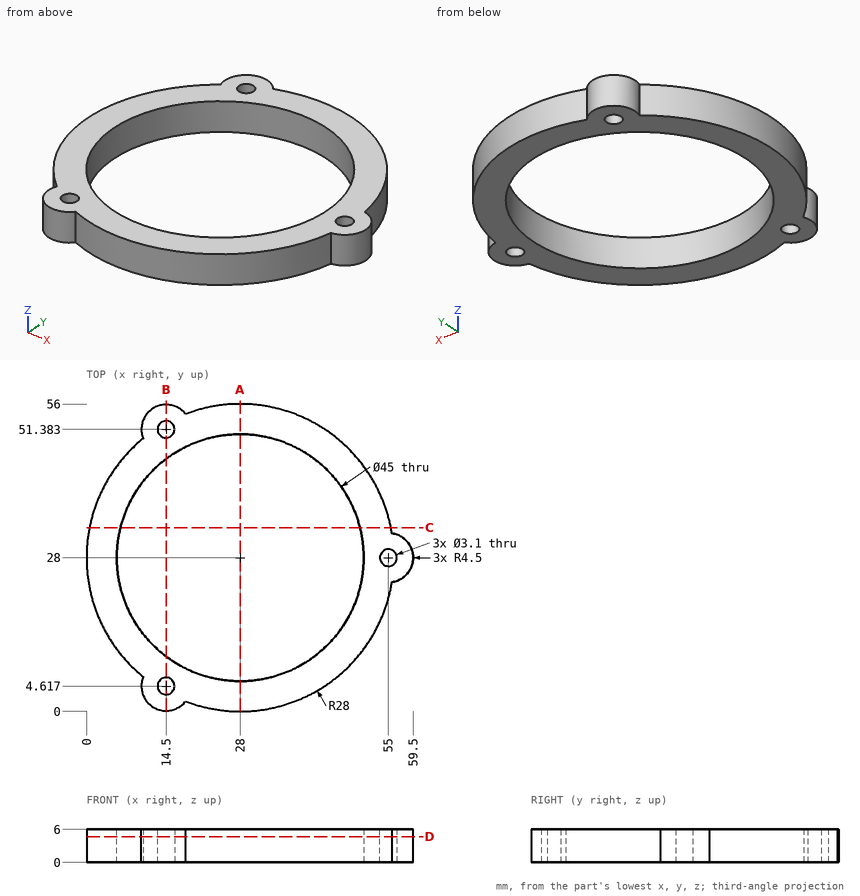
The figure shows three views and two pictorial views of one solid part (mm, origin at its lowest corner). Answer the questions. Give positions to 0.01 mm unless a question says otherwise; leave off trailing zeros. Write each loop counter-clockwise with the first axis right and the second up, starting at its lowest first coordinate (ties: lowest second). Pieces come first, ordered by that corner, then holes. Notation, with made-up numbers: M -17,43 L 35,43 A24 ccw 35,71 Z; hole C 1,-35 d11. An arc over 180 degrees is marked long. One line per item, written item: value. Start each with the question number.
(1) Find section A-A (x = 28). Determine the outline of the cut face in (y, z).
(2) Find section B-B (x = 14.5). Determine the outline of the cut face in (y, z).
(3) Find the intervals of material crossed by line 1 (Y direction, x = 14.5, z = 1.4); line 2 (Y direction, x = 15.5, z = 3.5); line 3 (X direction, y = 31, z = 0.45) (1 decimal), in increasing order.
(4) Flat-ended cylindrical pins translate along their axes: pin 1 Ø1.5 at (x, z) = (46.5, 1) entering from -Y (1 decimal); pin 2 Ø1.5 at (x, z) = (6.5, 1.5) entering from +Y. Find the tip coordinate at first contact, or state that the pin passes through.
(5) Find section C-C (y = 33.5). Determine the outline of the cut face in (x, z) (1 decimal).
(6) Find section D-D (z = 4.7). Give the number of separate pieces and of enclosed holes in the cut face.
Results below:
1. outline: M 0,0 L 5.5,0 L 5.5,6 L 0,6 Z; M 50.5,0 L 56,0 L 56,6 L 50.5,6 Z
2. outline: M 0.12,0 L 3.07,0 L 3.07,6 L 0.12,6 Z; M 6.17,0 L 10,0 L 10,6 L 6.17,6 Z; M 46,0 L 49.83,0 L 49.83,6 L 46,6 Z; M 52.93,0 L 55.88,0 L 55.88,6 L 52.93,6 Z
3. line 1: y = 0.12 to 3.07, 6.17 to 10, 46 to 49.83, 52.93 to 55.88
3. line 2: y = 0.23 to 3.43, 5.8 to 9.29, 46.71 to 50.2, 52.57 to 55.77
3. line 3: x = 0.2 to 5.7, 50.3 to 58.4
4. pin 1: stops at y = 6.3
4. pin 2: stops at y = 46.8
5. outline: M 0.5,0 L 6.2,0 L 6.2,6 L 0.5,6 Z; M 49.8,0 L 55.5,0 L 55.5,6 L 49.8,6 Z
6. separate pieces: 1
6. enclosed holes: 4
